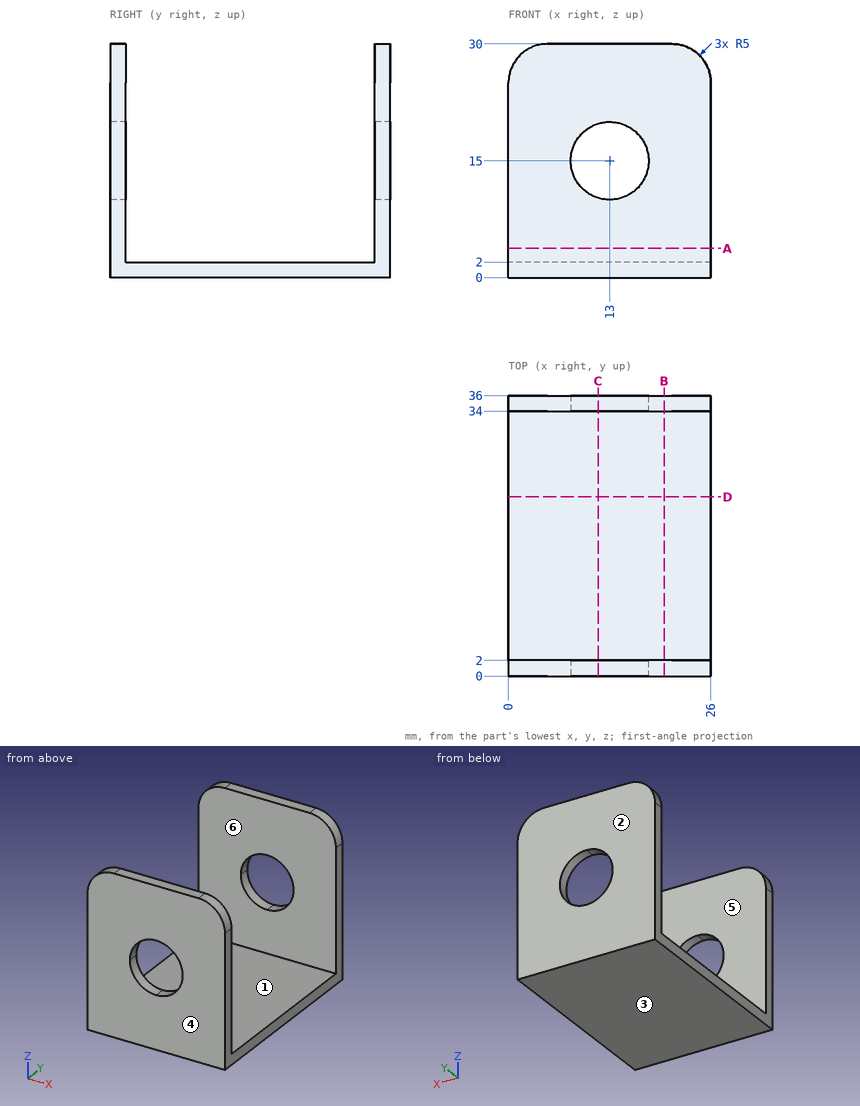
The drawing under review shows one solid part. Ordinate dimensions are in mm from its lowest x, y, z. A direction names the side the tool comes from. Round coordinates to 2 decimals unless told otherwise and drop trailing zeros. Write each loop counter-clockwise with the first axis right and the second up, starting at its lowest first coordinate (ties: lowest second). Pieces come first, ordered by that corner, then holes. Notation, with made-up numbers: (71, 76.5) - (96, 76.5) arc R11 cw to (96, 81.5) - close; hole circle Ø9 at (-25, 24.5). An arc over 180 degrees is marked (long way). Put each result on its own line as item: value.
Q1. We need section B-B (x = 20). Give the boundary of the cut face in (y, z).
Solved:
outline: (0, 0) - (36, 0) - (36, 30) - (34, 30) - (34, 2) - (2, 2) - (2, 30) - (0, 30) - close
Q2. Machinability: for the marked faces 1 and 2, which of the approach directions +Z, -Z, +X, -X, +Y, -Y give a long, thin tool a straight path to every point of the face, cutting with its end or side? Answer none if there is none.
Solved:
face 1: +Z, +X, -X
face 2: +Z, -Z, +X, -X, +Y
Q3. We need section D-D (y = 23). Give the boundary of the cut face in (x, z).
Solved:
outline: (0, 0) - (26, 0) - (26, 2) - (0, 2) - close
Q4. We need section C-C (x = 11.5). Give the boundary of the cut face in (y, z).
Solved:
outline: (0, 0) - (36, 0) - (36, 10.23) - (34, 10.23) - (34, 2) - (2, 2) - (2, 10.23) - (0, 10.23) - close; (0, 19.77) - (2, 19.77) - (2, 30) - (0, 30) - close; (34, 19.77) - (36, 19.77) - (36, 30) - (34, 30) - close
Q5. Wall thickness on probe 1 along Y at (x, z) = (7, 25.75); probe 2 along Z at (x, y) = (11.75, 28.5): over which ranges is each line inside the solid? List them lowest first.
Solved:
probe 1: y = 0 to 2, 34 to 36
probe 2: z = 0 to 2
Q6. Insertion check: pin 1 Ø1 at (y, z) = (25.5, 3.5) entering from +X; pin 2 Ø10 at (x, y) = (9.5, 11.5) entering from +Z. Each pin has a flat end and moves straight along its axis. Give the tip position at first contact, or say it passes through.
Solved:
pin 1: passes through
pin 2: stops at z = 2
Q7. We need section A-A (z = 3.75). Give the boundary of the cut face in (x, y), and give its area (3 significant figures).
Solved:
outline: (0, 0) - (26, 0) - (26, 2) - (0, 2) - close; (0, 34) - (26, 34) - (26, 36) - (0, 36) - close
area: 104 mm2
Q8. Mouldability with a two-part tool opening along Y and no side actions: class the marked faces 3, 4, 5 and 6 as released by +Y, released by -Y, zero draft, split by the parting line, or undercut.
Solved:
face 3: zero draft
face 4: released by -Y
face 5: undercut
face 6: undercut
